Design review of the part built by this model. Coordinates are the model's own, in mm. Coordinates: 2 decimals unless noted, no trailing zeros. Loops run counter-clockwise (first coordinate to the right, second up) from the corner with the lowest first, then second, coordinate; pieces in that order, holes last. Notation, with made-up numbers: (56, 77.25) -> (105, 77.25) arc R27 ccw to (105, 100.25) -> close; hole circle Ø11 at (-34, 16). An arc over 180 degrees is marked (long way). Use one line per item in the form item = value. Start each with the question number.
1. Consider section B-B (y = 0.35). State how many separate pieces and enclosed holes the cut face has, then the cut area to 3 significant figures.
2. For pin 1 (4 mm diameter, centred on x = -70, z = -90, fed in from -Y); pin 2 (0.5 mm diameter, centred on x = 12, y = 0.5, fed in from +Z), all flat-tipped, find the tip position at first contact; note any pin that passes through.
3. Consider section C-C (x = -70). State the section outline as (y, z) points.
4. Wall thickness on line 1 (Z direction, x = -85, y = 0.7); line 2 (Z direction, x = -70, y = 0.65); line 3 (Z direction, x = 70, y = 0.7): over which ranges is each line inside the solid? List them lowest first. Write a range as from..to.
5. Consider section A-A (x = 47.5). State the section outline as (y, z) points.
6. Consider section D-D (x = 69.5). State the section outline as (y, z) points, then the cut area to 3 significant figures.
from build123d import *

# Parameters (mm, degrees)
ESQUISSE1_R        = 1.5
ESQUISSE1_R_2      = 3.25
BOSS_EXTRU_1_DEPTH = 1


with BuildPart() as part:
    # Esquisse1 → Boss.-Extru.1 (new body)
    with BuildSketch(Plane(origin=(0, 0, 0), x_dir=(1, 0, 0), z_dir=(0, 1, 0))):
        Polygon((-40, 100), (-40, 75), (40, 75), (40, 100), (100, 100), (100, 55), (-50, 55), (-50, -55), (100, -55), (100, -100), (40, -100), (40, -75), (-40, -75), (-40, -100), (-100, -100), (-100, 100), align=None)
        with Locations((-85, 90)):
            Circle(ESQUISSE1_R, mode=Mode.SUBTRACT)
        with Locations((-55, 90)):
            Circle(ESQUISSE1_R, mode=Mode.SUBTRACT)
        with Locations((-55, -90)):
            Circle(ESQUISSE1_R, mode=Mode.SUBTRACT)
        with Locations((-85, -90)):
            Circle(ESQUISSE1_R, mode=Mode.SUBTRACT)
        with Locations((55, -90)):
            Circle(ESQUISSE1_R, mode=Mode.SUBTRACT)
        with Locations((85, -90)):
            Circle(ESQUISSE1_R, mode=Mode.SUBTRACT)
        with Locations((-55, -58)):
            Circle(ESQUISSE1_R, mode=Mode.SUBTRACT)
        with Locations((-55, -40)):
            Circle(ESQUISSE1_R, mode=Mode.SUBTRACT)
        with Locations((-55, 40)):
            Circle(ESQUISSE1_R, mode=Mode.SUBTRACT)
        with Locations((-55, 58)):
            Circle(ESQUISSE1_R, mode=Mode.SUBTRACT)
        with Locations((-70, -90)):
            Circle(ESQUISSE1_R_2, mode=Mode.SUBTRACT)
        with Locations((70, -90)):
            Circle(ESQUISSE1_R_2, mode=Mode.SUBTRACT)
        with Locations((70, 90)):
            Circle(ESQUISSE1_R_2, mode=Mode.SUBTRACT)
        with Locations((-70, 90)):
            Circle(ESQUISSE1_R_2, mode=Mode.SUBTRACT)
        with Locations((55, 90)):
            Circle(ESQUISSE1_R, mode=Mode.SUBTRACT)
        with Locations((85, 90)):
            Circle(ESQUISSE1_R, mode=Mode.SUBTRACT)
    extrude(amount=BOSS_EXTRU_1_DEPTH)


solid = part.part
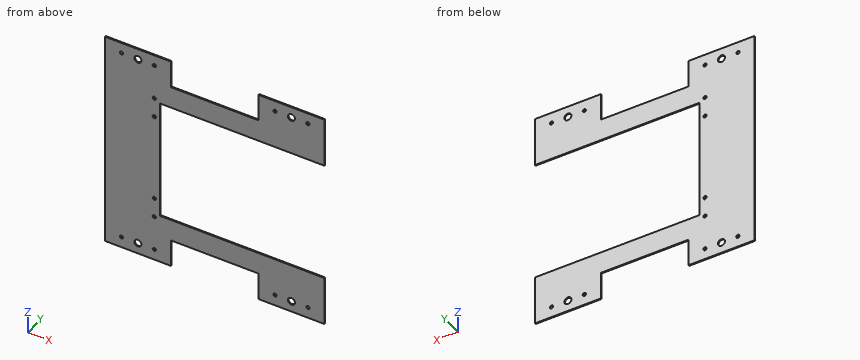
Geometry check:
q1.separate_pieces = 1
q1.enclosed_holes = 16
q1.area = 19,300 mm²
q2.pin_1 = through
q2.pin_2 = 75
q3.outline = (0, -100) -> (1, -100) -> (1, -93.25) -> (0, -93.25) -> close; (0, -86.75) -> (1, -86.75) -> (1, 86.75) -> (0, 86.75) -> close; (0, 93.25) -> (1, 93.25) -> (1, 100) -> (0, 100) -> close
q4.line_1 = -100..-91.5, -88.5..88.5, 91.5..100
q4.line_2 = -100..-93.25, -86.75..86.75, 93.25..100
q4.line_3 = -100..-93.25, -86.75..-55, 55..86.75, 93.25..100
q5.outline = (0, -100) -> (1, -100) -> (1, -55) -> (0, -55) -> close; (0, 55) -> (1, 55) -> (1, 100) -> (0, 100) -> close
q6.outline = (0, -100) -> (1, -100) -> (1, -93.21) -> (0, -93.21) -> close; (0, -86.79) -> (1, -86.79) -> (1, -55) -> (0, -55) -> close; (0, 55) -> (1, 55) -> (1, 86.79) -> (0, 86.79) -> close; (0, 93.21) -> (1, 93.21) -> (1, 100) -> (0, 100) -> close
q6.area = 77.2 mm²
